Autodesk Fusion 360 part; units mm, degrees
sketch "Sketch1" plane through (0, 0, 0) normal (0, 0, 1) x (1, 0, 0)
  line L0 (40, -40) -> (-60, -40)
  line L1 (-60, -40) -> (-60, 60)
  line L2 (-60, 60) -> (40, 60)
  line L3 (40, 60) -> (40, -40)
  dimension "d1" = 100
  dimension "d2" = 100
extrude "Extrude1" add sketch "Sketch1" along normal blind 2.5
sketch "Sketch2" plane through (0, 0, 2.5) normal (0, 0, 1) x (-1, 0, 0)
  line L0 (-40, -60) -> (60, -60)
  line L1 (60, -60) -> (60, 40)
  line L2 (60, 40) -> (-40, 40)
  line L3 (-40, 40) -> (-40, -60)
  point P0 (44.5, -10)
  point P1 (38, 36.5)
  point P2 (10, 36.5)
  point P3 (-18, 36.5)
  point P4 (-24.5, -10)
  point P5 (38, -56.5)
  point P6 (10, -56.5)
  point P7 (-18, -56.5)
  dimension "d7" = 50
  dimension "d11" = 50
  dimension "d12" = 28
  dimension "d13" = 28
  dimension "d14" = 3.5
  dimension "d15" = 3.5
  dimension "d16" = 3.5
  dimension "d17" = 50
  dimension "d25" = 50
  dimension "d26" = 28
  dimension "d27" = 28
  dimension "d28" = 3.5
  dimension "d29" = 3.5
  dimension "d30" = 3.5
  dimension "d34" = 15.5
  dimension "d35" = 15.5
hole "Hole1" at (-38, 56.5, 2.5) at (18, 56.5, 2.5) at (18, -36.5, 2.5) at (-38, -36.5, 2.5) direction (0, 0, -1) diameter 3 depth 10 tip angle 118
sketch "Sketch3" plane through (0, 0, 2.5) normal (0, 0, 1) x (-1, 0, 0)
  circle A0 centre (-18, 36.5) radius 1.5
  circle A1 centre (38, -56.5) radius 1.5
  circle A2 centre (-18, -56.5) radius 1.5
  circle A3 centre (38, 36.5) radius 1.5
  line L0 (-40, -60) -> (60, -60)
  line L1 (60, -60) -> (60, 40)
  line L2 (60, 40) -> (-40, 40)
  line L3 (-40, 40) -> (-40, -60)
  circle A4 centre (10, -10) radius 7.5
  dimension "d36" = 15
extrude "Extrude2" cut sketch "Sketch3" against normal blind 2.5 contours A4
sketch "Sketch4" plane through (0, 0, 0) normal (0, 0, 1) x (1, 0, 0)
  circle A0 centre (-10, 10) radius 15
  circle A1 centre (-10, 10) radius 7.5
  circle A2 centre (-10, 21.25) radius 1.5
  circle A3 centre (-2.045, 17.955) radius 1.5
  circle A4 centre (1.25, 10) radius 1.5
  circle A5 centre (-2.045, 2.045) radius 1.5
  circle A6 centre (-10, -1.25) radius 1.5
  circle A7 centre (-17.955, 2.045) radius 1.5
  circle A8 centre (-21.25, 10) radius 1.5
  circle A9 centre (-17.955, 17.955) radius 1.5
  point P0 (-10, 21.25)
  point P1 (-17.955, 17.955)
  point P2 (-21.25, 10)
  point P3 (-17.955, 2.045)
  point P4 (-10, -1.25)
  point P5 (-2.045, 2.045)
  point P6 (1.25, 10)
  point P7 (-2.045, 17.955)
  point P8 (-17.955, 17.955)
  point P9 (-21.25, 10)
  point P10 (-17.955, 2.045)
  point P11 (-10, -1.25)
  point P12 (-2.045, 2.045)
  point P13 (1.25, 10)
  point P14 (-2.045, 17.955)
  dimension "d39" = 30
  dimension "d40" = 11.25
  dimension "d42" = 360
  dimension "d46" = 3
  dimension "d47" = 3
  dimension "d48" = 3
  dimension "d49" = 3
  dimension "d50" = 3
  dimension "d51" = 3
  dimension "d52" = 3
  dimension "d53" = 3
extrude "Extrude3" cut sketch "Sketch4" along normal blind 9 contours A2 | A3 | A4 | A5 | A6 | A7 | A8 | A9
sketch "Sketch7" plane through (0, 0, 2.5) normal (0, 0, 1) x (-1, 0, 0)
  circle A0 centre (10, -21.25) radius 1.5
  circle A1 centre (10, 1.25) radius 1.5
  circle A2 centre (2.045, -2.045) radius 1.5
  circle A3 centre (17.955, -17.955) radius 1.5
  circle A4 centre (2.045, -17.955) radius 1.5
  circle A5 centre (17.955, -2.045) radius 1.5
  circle A6 centre (-1.25, -10) radius 1.5
  circle A7 centre (21.25, -10) radius 1.5
  circle A8 centre (10, -10) radius 7.5
  circle A9 centre (-18, 36.5) radius 1.5
  circle A10 centre (38, -56.5) radius 1.5
  circle A11 centre (-18, -56.5) radius 1.5
  circle A12 centre (38, 36.5) radius 1.5
  line L0 (-40, -60) -> (60, -60)
  line L1 (60, -60) -> (60, 40)
  line L2 (60, 40) -> (-40, 40)
  line L3 (-40, 40) -> (-40, -60)
  circle A13 centre (10, -10) radius 15
  dimension "d56" = 30
sketch "Sketch8" plane through (0, 0, 2.5) normal (0, 0, 1) x (-1, 0, 0)
  line L0 (10, -10) -> (10, 40)
  line L1 (10, 40) -> (10, -60)
sketch "Sketch9" plane through (0, 0, 2.5) normal (0, 0, 1) x (-1, 0, 0)
  line L0 (-40, -10) -> (60, -10)
sketch "Sketch10" plane through (0, 0, 2.5) normal (0, 0, 1) x (-1, 0, 0)
  line L0 (-40, 40) -> (60, -60)
sketch "Sketch11" plane through (0, 0, 0) normal (0, 0, 1) x (1, 0, 0)
  line L0 (-60, -40) -> (40, 60)
sketch "Sketch13" plane through (0, 0, 2.5) normal (0, 0, 1) x (-1, 0, 0)
  line L0 (-17.6512, 30) -> (4, 30)
  line L1 (5, 29) -> (5, 6.4828)
  line L2 (3.2792, 5.7897) -> (-18.372, 28.3069)
  arc A0 (-17.6512, 30) -> (-18.372, 28.3069) centre (-17.6512, 29) ccw
  arc A1 (5, 29) -> (4, 30) centre (4, 29) ccw
  arc A2 (3.2792, 5.7897) -> (5, 6.4828) centre (4, 6.4828) ccw
  line L3 (-40, 40) -> (60, -60)
  arc A3 (-6.4828, -5) -> (-5.7897, -3.2792) centre (-6.4828, -4) ccw
  line L4 (-29, -5) -> (-6.4828, -5)
  line L5 (-5.7897, -3.2792) -> (-28.3069, 18.372)
  arc A4 (-28.3069, 18.372) -> (-30, 17.6512) centre (-29, 17.6512) ccw
  line L6 (-30, 17.6512) -> (-30, -4)
  arc A5 (-30, -4) -> (-29, -5) centre (-29, -4) ccw
  line L7 (-40, -10) -> (60, -10)
  line L8 (-29, -15) -> (-6.4828, -15)
  arc A6 (-5.7897, -16.7208) -> (-6.4828, -15) centre (-6.4828, -16) ccw
  line L9 (-5.7897, -16.7208) -> (-28.3069, -38.372)
  arc A7 (-30, -37.6512) -> (-28.3069, -38.372) centre (-29, -37.6512) ccw
  line L10 (-30, -37.6512) -> (-30, -16)
  arc A8 (-29, -15) -> (-30, -16) centre (-29, -16) ccw
  line L11 (60, 40) -> (-40, -60)
  line L12 (5, -49) -> (5, -26.4828)
  arc A9 (4, -50) -> (5, -49) centre (4, -49) ccw
  arc A10 (5, -26.4828) -> (3.2792, -25.7897) centre (4, -26.4828) ccw
  line L13 (3.2792, -25.7897) -> (-18.372, -48.3069)
  line L14 (-17.6512, -50) -> (4, -50)
  arc A11 (-18.372, -48.3069) -> (-17.6512, -50) centre (-17.6512, -49) ccw
  line L15 (10, 40) -> (10, -60)
  arc A12 (16.7208, -25.7897) -> (15, -26.4828) centre (16, -26.4828) ccw
  line L16 (15, -49) -> (15, -26.4828)
  line L17 (16.7208, -25.7897) -> (38.372, -48.3069)
  line L18 (37.6512, -50) -> (16, -50)
  arc A13 (15, -49) -> (16, -50) centre (16, -49) ccw
  arc A14 (37.6512, -50) -> (38.372, -48.3069) centre (37.6512, -49) ccw
  arc A15 (26.4828, -15) -> (25.7897, -16.7208) centre (26.4828, -16) ccw
  line L19 (25.7897, -16.7208) -> (48.3069, -38.372)
  line L20 (49, -15) -> (26.4828, -15)
  arc A16 (50, -16) -> (49, -15) centre (49, -16) ccw
  line L21 (50, -37.6512) -> (50, -16)
  arc A17 (48.3069, -38.372) -> (50, -37.6512) centre (49, -37.6512) ccw
  line L22 (25.7897, -3.2792) -> (48.3069, 18.372)
  arc A18 (50, 17.6512) -> (48.3069, 18.372) centre (49, 17.6512) ccw
  line L23 (50, 17.6512) -> (50, -4)
  arc A19 (49, -5) -> (50, -4) centre (49, -4) ccw
  line L24 (49, -5) -> (26.4828, -5)
  arc A20 (25.7897, -3.2792) -> (26.4828, -5) centre (26.4828, -4) ccw
  line L25 (37.6512, 30) -> (16, 30)
  arc A21 (38.372, 28.3069) -> (37.6512, 30) centre (37.6512, 29) ccw
  line L26 (16.7208, 5.7897) -> (38.372, 28.3069)
  arc A22 (15, 6.4828) -> (16.7208, 5.7897) centre (16, 6.4828) ccw
  line L27 (15, 29) -> (15, 6.4828)
  arc A23 (16, 30) -> (15, 29) centre (16, 29) ccw
  point P0 (-20, 30)
  point P1 (5, 30)
  point P2 (5, 4)
  dimension "d57" = 1
extrude "Extrude7" cut sketch "Sketch13" against normal blind 5
sketch "Sketch14" plane through (0, 60, 0) normal (0, 1, 0) x (-1, 0, 0)
  line L0 (-40, 0) -> (60, 0)
  line L1 (60, 0) -> (60, 2.5)
  line L2 (60, 2.5) -> (-40, 2.5)
  line L3 (-40, 2.5) -> (-40, 0)
  line L4 (-40, 2.5) -> (-37.5, 0)
  point P0 (-40, 2.5)
  point P1 (-40, 0)
  point P2 (-37.5, 0)
  point P3 (-40, 0)
  dimension "d60" = 2.5
extrude "Extrude5" cut sketch "Sketch14" against normal blind 104 contours L0 L3 L4
sketch "Sketch15" plane through (0, 60, 0) normal (0, 1, 0) x (-1, 0, 0)
  line L0 (-40, 2.5) -> (-37.5, 0)
  line L1 (-37.5, 0) -> (60, 0)
  line L2 (60, 0) -> (60, 2.5)
  line L3 (60, 2.5) -> (-40, 2.5)
  line L4 (60, 2.5) -> (57.5, 0)
  point P0 (60, 2.5)
  point P1 (60, 0)
  point P2 (57.5, 0)
  point P3 (60, 0)
  dimension "d63" = 2.5
extrude "Extrude6" cut sketch "Sketch15" against normal blind 105 contours L1 L2 L4
sketch "Sketch16" plane through (0, 0, 2.5) normal (0, 0, 1) x (-1, 0, 0)
sketch "Sketch17" plane through (0, 0, 2.5) normal (0, 0, 1) x (-1, 0, 0)
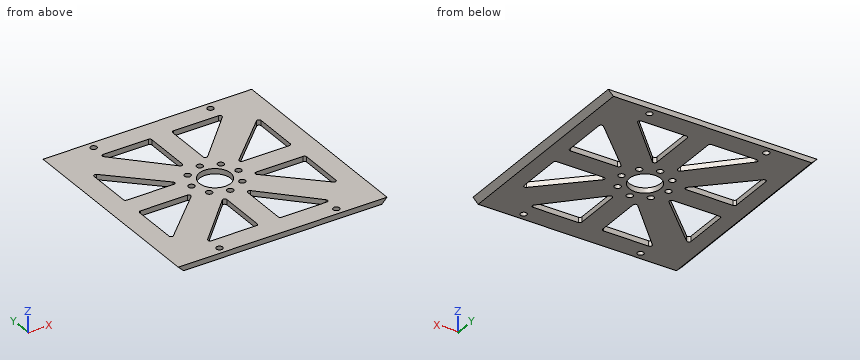
Can you work these out from the model? Positions are in its coordinate system, mm. Round coordinates to 2 decimals unless told otherwise and drop trailing zeros. Write each loop counter-clockwise with the first axis right and the second up, starting at its lowest first coordinate (ties: lowest second). Pieces come first, ordered by that corner, then holes. Notation, with made-up numbers: (62, 80) -> (81, 80) arc R21 cw to (81, 109) -> close; hole circle Ø4 at (40.5, 72.25). An arc over 180 degrees is marked (long way). One line per question, with ' | ' between items. Start each with the question number.
1) Suppose I cut it at D-D on y = 29. Write out the boundary of the cut face in (x, z).
2) I'm going to push flat-ended pins straight in: P1, Ø1.5, axis at y = 37, z = 1, coming from the -X side; P2, Ø2.5, axis at x = 18, y = -36.5, coming from the +Z side; P3, Ø1, axis at y = -18, z = 1, coming from the -X side; P4, Ø5, axis at x = -17.955, y = 17.955, coming from the +Z side. Where does each tip first touch, or does it pass through?
3) Suppose I cut it at B-B on x = -10. Write out the boundary of the cut face in (y, z).
4) Suppose I cut it at A-A on y = 56.5. Write out the boundary of the cut face in (x, z).
5) I need wall thicknesses on line 1 (Y direction, x = -10, z = 1.25); line 2 (Y direction, x = 12, z = 0.25); line 3 (X direction, y = 56.5, z = 1.7). Which ranges of each line are inside material? Lowest first, please. Write a range as [from, to].
6) Suppose I cut it at C-C on x = -44.5. Write out the boundary of the cut face in (y, z).
Return value:
1) outline: (-60, 2.5) -> (-57.5, 0) -> (-50, 0) -> (-50, 2.5) -> close; (-38.56, 0) -> (-19.81, 0) -> (-19.81, 2.5) -> (-38.56, 2.5) -> close; (-15, 0) -> (-5, 0) -> (-5, 2.5) -> (-15, 2.5) -> close; (-0.19, 0) -> (18.56, 0) -> (18.56, 2.5) -> (-0.19, 2.5) -> close; (30, 0) -> (37.5, 0) -> (40, 2.5) -> (30, 2.5) -> close
2) P1: stops at x = -59.25 | P2: passes through | P3: stops at x = -59 | P4: stops at z = 2.5
3) outline: (-40, 0) -> (-2.75, 0) -> (-2.75, 2.5) -> (-40, 2.5) -> close; (0.25, 0) -> (2.5, 0) -> (2.5, 2.5) -> (0.25, 2.5) -> close; (17.5, 0) -> (19.75, 0) -> (19.75, 2.5) -> (17.5, 2.5) -> close; (22.75, 0) -> (60, 0) -> (60, 2.5) -> (22.75, 2.5) -> close
4) outline: (-60, 2.5) -> (-57.5, 0) -> (-39.5, 0) -> (-39.5, 2.5) -> close; (-36.5, 0) -> (16.5, 0) -> (16.5, 2.5) -> (-36.5, 2.5) -> close; (19.5, 0) -> (37.5, 0) -> (40, 2.5) -> (19.5, 2.5) -> close
5) line 1: y = [-40, -2.75], [0.25, 2.5], [17.5, 19.75], [22.75, 60] | line 2: y = [-40, -30], [-21.68, -2.69], [5, 15], [22.69, 41.68], [50, 60] | line 3: x = [-59.2, -39.5], [-36.5, 16.5], [19.5, 39.2]
6) outline: (-40, 0) -> (-14.71, 0) -> (-14.71, 2.5) -> (-40, 2.5) -> close; (5, 0) -> (15, 0) -> (15, 2.5) -> (5, 2.5) -> close; (34.71, 0) -> (60, 0) -> (60, 2.5) -> (34.71, 2.5) -> close
